from build123d import *

# Parameters (mm, degrees)
ESQUISSE1_R                  = 125
ESQUISSE1_W                  = 40.2
ESQUISSE1_H                  = 20.2
ESQUISSE1_W_2                = 18.123947537
ESQUISSE1_H_2                = 28.637153683
BOSS_EXTRU_1_DEPTH           = 15
ENL_V_MAT_EXTRU_1_DEPTH      = 15
R_P_TITION_CIRCULAIRE1_COUNT = 4


with BuildPart() as part:
    # Esquisse1 → Boss.-Extru.1 (new body)
    with BuildSketch(Plane.XY):
        Circle(ESQUISSE1_R)
        with Locations((10.6, 0)):
            Rectangle(ESQUISSE1_W, ESQUISSE1_H, mode=Mode.SUBTRACT)
        with Locations((-0.438026231, 37.232201346)):
            Rectangle(ESQUISSE1_W_2, ESQUISSE1_H_2, mode=Mode.SUBTRACT)
    extrude(amount=BOSS_EXTRU_1_DEPTH)

    # Esquisse3 → Enlèv. mat.-Extru.1 (cut)
    with BuildSketch(Plane.XY.offset(15)):
        Polygon((112.62821071, -84.343939462), (92.432755834, -64.148484587), (64.148484587, -92.432755834), (84.343939462, -112.62821071), align=None)
        Polygon((81.950288575, -89.021356387), (89.021356387, -81.950288575), (39.271363502, -32.20029569), (32.20029569, -39.271363502), align=None)
        Polygon((53.431679247, -67.573814871), (67.573814871, -53.431679247), (61.916960621, -47.774824997), (47.774824997, -61.916960621), align=None)
    enl_v_mat_extru_1 = extrude(amount=-ENL_V_MAT_EXTRU_1_DEPTH, mode=Mode.SUBTRACT)

    # Répétition circulaire1: Enlèv. mat.-Extru.1 ×4 about axis
    r_p_tition_circulaire1_axis = Axis((0, 0, 0), (0, 0, 1))
    for i in range(1, R_P_TITION_CIRCULAIRE1_COUNT):
        add(enl_v_mat_extru_1.rotate(r_p_tition_circulaire1_axis, i * 360 / R_P_TITION_CIRCULAIRE1_COUNT), mode=Mode.SUBTRACT)


solid = part.part
Build history of the part. All positions in model axes, mm. A direction names the side the tool comes from. Round coordinates to 2 decimals unless told otherwise and drop trailing zeros. Order: outer loops, then holes, each group sorted by start corner. A loop starts at its lowest first (then second) coordinate and runs counter-clockwise, first axis right, second up. Notation, with made-up numbers: M 66.5,81 L 89.5,81 A22 ccw 89.5,110 Z; hole C 55.5,28 d5. An arc over 180 degrees is marked long. Use CSV: the item, a comma, the result in double quotes. Start each with the question number.
(1) Cut at D-D on y = 98. List the corners of the cut face in (x, z), then the cut area to 3 significant figures.
(2) Drill centre lines: probe 1 along Y at (x, z) = (-74, 7); probe 2 along X at (y, z) = (57, 2.5); probe 3 along X at (y, z) = (42, 10.5). Where is each one in solid material? Low to high.
(3) Tool access for faces 4 (the face through (-50.64, -64.78, 7.6)), 5 (the face through (-68.691, -96.975, 7.605)), 6 (the face through (68.565, -96.85, 7.605)): list every direction of +Z, -Z, +X, -X, +Y, -Y with a clear straight run to the whole face (end or side of a thin tool).
(4) Cut at C-C on x = -27.5. List the corners of the cut face in (y, z).
(5) Cut at A-A on y = -1.5. List the corners of the cut face in (x, z).
(6) Cut at B-B on z = 3. State how many separate pieces and enclosed holes the cut face has, then the cut area to 3 significant figures.
(7) Mould opens along Y. For faces 1 (the face through (-68.565, 96.85, 7.605)), 2 (the face through (-124.995, 1.093, 7.395)), 3 (the face through (-1.093, -124.995, 7.395)) say: +Y half, -Y half, draft (parallel to the pull), parting line (faces both ways), or undercut.
(8) Flat gauge pins, fed straight in: P1, Ø4.5, axis at x = 17.5, z = 10.5, coming from the -Y side; P2, Ø8, axis at y = 16.5, z = 9.5, coming from the -X side; P3, Ø1.5, axis at x = 55.5, z = 5, coming from the -Y side. Where does each tip first touch, or does it go through?
Findings:
1,outline,"M -69.72,0 L 69.72,0 L 69.72,15 L -69.72,15 Z"
1,area,"2,090 mm^2"
2,probe 1,"y = -82.58 to -81.07, -66.93 to 66.93, 81.07 to 82.58"
2,probe 2,"x = -111.25 to -64.07, -49.93 to 49.93, 64.07 to 111.25"
2,probe 3,"x = -117.73 to -49.07, -34.93 to -9.5, 8.62 to 34.93, 49.07 to 117.73"
3,face 4,"+Z, -Z"
3,face 5,"+Z, -Z, -X"
3,face 6,"+Z, -Z, +X"
4,outline,"M -121.94,0 L 121.94,0 L 121.94,15 L -121.94,15 Z"
5,outline,"M -124.99,0 L -9.5,0 L -9.5,15 L -124.99,15 Z; M 30.7,0 L 124.99,0 L 124.99,15 L 30.7,15 Z"
6,separate pieces,"1"
6,enclosed holes,"2"
6,area,"42,800 mm^2"
7,face 1,"undercut"
7,face 2,"parting line"
7,face 3,"-Y half"
8,P1,"stops at y = -124.07"
8,P2,"stops at x = -124.37"
8,P3,"stops at y = -112.37"
